Here's how the part is built. I have some questions about the finished solid (model axes, mm). A direction names the side the tool comes from. Round coordinates to 2 decimals unless told otherwise and drop trailing zeros. Order: outer loops, then holes, each group sorted by start corner. A loop starts at its lowest first (then second) coordinate and runs counter-clockwise, first axis right, second up. Notation, with made-up numbers: (0.25, 58.5) -> (11.25, 58.5) arc R30 cw to (11.25, 93.5) -> close; hole circle Ø6 at (33, 23.5). An arc over 180 degrees is marked (long way). Use a Markdown table: item, result. Add a question column.
from build123d import *

# Parameters (mm, degrees)
SKETCH1_R           = 1.5
BOSS_EXTRUDE1_DEPTH = 2.5


with BuildPart() as part:
    # Sketch1 → Boss-Extrude1 (new, symmetric)
    with BuildSketch(Plane.XY):
        with BuildLine():
            Line((-24.78125, 50), (24.78125, 50))
            ThreePointArc((24.78125, 50), (27.28125, 47.5), (24.78125, 45))
            Line((24.78125, 45), (2.5, 45))
            Line((2.5, 45), (2.5, -45))
            Line((2.5, -45), (22.5, -45))
            Line((22.5, -45), (22.5, -50))
            Line((22.5, -50), (-22.5, -50))
            Line((-22.5, -50), (-22.5, -45))
            Line((-22.5, -45), (-2.5, -45))
            Line((-2.5, -45), (-2.5, 45))
            Line((-2.5, 45), (-24.78125, 45))
            ThreePointArc((-24.78125, 45), (-27.28125, 47.5), (-24.78125, 50))
        make_face()
        with Locations((-24.78125, 47.5)):
            Circle(SKETCH1_R, mode=Mode.SUBTRACT)
        with Locations((24.78125, 47.5)):
            Circle(SKETCH1_R, mode=Mode.SUBTRACT)
    extrude(amount=BOSS_EXTRUDE1_DEPTH, both=True)


solid = part.part
(1) I'm going to push flat-ended pins straight in: P1, Ø1.5, axis at y = -47.5, z = -1, coming from the +X side; P2, Ø1.5, axis at y = -48, z = -1, coming from the -X side; P3, Ø1.5, axis at y = 9.5, z = 1, coming from the +X side. Where does each tip first touch, or does it pass through?
(2) I want a section at A-A on x = 13. List the corners of the cut face in (y, z) for me.
(3) I want a section at D-D on y = -37.5. List the corners of the cut face in (x, z) for me.
(4) If we mould it in two halves opening along Y, with no side actions, what happens to faces 1 (the cylindrical face through (27.28, 47.55, 0.04)), 2 (the flat face through (-22.5, -48, 0)), 3 (the flat face through (-13, 45, 0))? For each: pulls with the +Y half, pulls with the -Y half, needs draft (parallel to the pull), parting line crosses it, or undercut.
(5) On a 3-axis mill with a long thin cutter (end or side, diameter ignored), from which of +Z, -Z, +X, -X, +Y, -Y can I reach the whole of each face in a straight line? I mean faces 4 (the cylindrical face through (24.456, 46.036, -0.035)), 5 (the flat face through (-13, -45, 0)), 6 (the flat face through (14, 45, 0)), 7 (the flat face through (22.5, -47, 0)), 8 (the flat face through (0, 50, 0)). Say none if no direction works.
(6) I want a section at B-B on y = 47.5. List the corners of the cut face in (x, z) for me.
(7) I want a section at C-C on z = 1.7. List the corners of the cut face in (x, y) for me.
(8) Please list where these lines run through material, in increasing order: probe 1 along Y at (x, z) = (14.5, -1.55); probe 2 along X at (y, z) = (-20, 2.35). Write a range as from..to.
Output:
| question | item | result |
|---|---|---|
| 1 | P1 | x = 22.5 |
| 1 | P2 | x = -22.5 |
| 1 | P3 | x = 2.5 |
| 2 | outline | (-50, -2.5) -> (-45, -2.5) -> (-45, 2.5) -> (-50, 2.5) -> close; (45, -2.5) -> (50, -2.5) -> (50, 2.5) -> (45, 2.5) -> close |
| 3 | outline | (-2.5, -2.5) -> (2.5, -2.5) -> (2.5, 2.5) -> (-2.5, 2.5) -> close |
| 4 | face 1 | parting line crosses it |
| 4 | face 2 | needs draft |
| 4 | face 3 | undercut |
| 5 | face 4 | +Z, -Z |
| 5 | face 5 | +Z, -Z, -X |
| 5 | face 6 | +Z, -Z, +X |
| 5 | face 7 | +Z, -Z, +X, -Y |
| 5 | face 8 | +Z, -Z, +X, -X, +Y |
| 6 | outline | (-27.28, -2.5) -> (-26.28, -2.5) -> (-26.28, 2.5) -> (-27.28, 2.5) -> close; (-23.28, -2.5) -> (23.28, -2.5) -> (23.28, 2.5) -> (-23.28, 2.5) -> close; (26.28, -2.5) -> (27.28, -2.5) -> (27.28, 2.5) -> (26.28, 2.5) -> close |
| 7 | outline | (-24.78, 45) -> (-2.5, 45) -> (-2.5, -45) -> (-22.5, -45) -> (-22.5, -50) -> (22.5, -50) -> (22.5, -45) -> (2.5, -45) -> (2.5, 45) -> (24.78, 45) arc R2.5 ccw to (24.78, 50) -> (-24.78, 50) arc R2.5 ccw to start; hole circle Ø3 at (-24.78, 47.5); hole circle Ø3 at (24.78, 47.5) |
| 8 | probe 1 | -50..-45, 45..50 |
| 8 | probe 2 | -2.5..2.5 |
